```python
from build123d import *

# Parameters (mm, degrees)
F0_W     = 25
F0_H     = 16
F1_DEPTH = 4
F3_D     = 4.2
F3_DEPTH = 14.4
F3_TIP   = 1.2618073
F5_D     = 2.4
F5_DEPTH = 9.8
F5_TIP   = 0.7210327428


with BuildPart() as f1:
    # F0 (on Front) → F1 (new body, symmetric)
    with BuildSketch(Plane.XZ):
        Rectangle(F0_W, F0_H)
    extrude(amount=F1_DEPTH, both=True)

    # F3
    with Locations(Plane.XZ.offset(4)):
        with Locations((4.5, 2)):
            Hole(F3_D / 2, depth=F3_DEPTH)
            with Locations((0, 0, -(F3_DEPTH + F3_TIP / 2))):  # 118° drill point
                Cone(0, F3_D / 2, F3_TIP, mode=Mode.SUBTRACT)

    # F5
    with Locations(Plane.XY.offset(8)):
        with Locations((-0.5, 0), (-7.5, 0)):
            Hole(F5_D / 2, depth=F5_DEPTH)
            with Locations((0, 0, -(F5_DEPTH + F5_TIP / 2))):  # 118° drill point
                Cone(0, F5_D / 2, F5_TIP, mode=Mode.SUBTRACT)


solid = f1.part
```
Work out the finished part from the listing and answer in its coordinate system (mm). A direction names the side the tool comes from. Round coordinates to 2 decimals unless told otherwise and drop trailing zeros. Write each loop counter-clockwise with the first axis right and the second up, starting at its lowest first coordinate (ties: lowest second). Pieces come first, ordered by that corner, then holes. Notation, with made-up numbers: (0, -32.75) - (11, -32.75) arc R29 ccw to (11, -4.75) - close; hole circle Ø11 at (-27.75, 7). An arc over 180 degrees is marked (long way). Return JSON: item names as keys, results as strings. Group by question number.
Q1. The part is cut by section C-C on y = -2. Write down the section's boundary in (x, z), then the cut area to 3 significant figures.
Q2. The mould has two halves that part along X. Classify faces 3 (the flat face through (0, 4, 0)), 4 (the flat face through (12.5, 0, 0)), 5 (the cylindrical face through (4.96, 0.06, -0.05)), 6 (the conical face through (-0.665, -0.127, -2.396)): released by +X, released by -X, zero draft, split by the parting line, or undercut.
Q3. Find the intervals of material crossed by L1, parallel to X at y = 0, z = 1.25; L2, parallel to X at y = 0, z = 1.75; L3, parallel to Y at x = -7.5, z = 5, in increasing order.
Q4. The part is cut by section A-A on z = 2. Write down the section's boundary in (x, y).
Q5. For faces 1 (the flat face through (0, 2, 8)), 2 (the cylindrical face through (0.7, 0.05, 3.03)), determine the directions among +Z, -Z, +X, -X, +Y, -Y from which every point of the face is accessible in a straight line to the end or side of a thin tool.
Q6. The part is cut by section D-D on z = -0.75. Write down the section's boundary in (x, y), then the cut area to 3 significant figures.
Q7. Each of these flat-tipped pins is pushed along its axis until it touches: pin 1 Ø3.5 at (x, z) = (4.5, 2) entering from +Y; pin 2 Ø2 at (x, z) = (3, 2) entering from +Y. Where does it stop, or does it pass through?
Q8. The part is cut by section B-B on x = 4.5. Write down the section's boundary in (y, z), then the cut area to 3 significant figures.
Solved:
{
 "1": {"outline": "(-12.5, -8) - (12.5, -8) - (12.5, 8) - (-12.5, 8) - close; hole circle Ø4.2 at (4.5, 2)", "area": "386 mm²"},
 "2": {"face 3": "zero draft", "face 4": "released by +X", "face 5": "undercut", "face 6": "undercut"},
 "3": {"L1": "-12.5 to -8.7, -6.3 to -1.7, 0.7 to 2.54, 6.46 to 12.5", "L2": "-12.5 to -8.7, -6.3 to -1.7, 0.7 to 2.41, 6.59 to 12.5", "L3": "-4 to -1.2, 1.2 to 4"},
 "4": {"outline": "(-12.5, -4) - (2.4, -4) - (2.4, 4) - (-12.5, 4) - close; (6.6, -4) - (12.5, -4) - (12.5, 4) - (6.6, 4) - close; hole circle Ø2.4 at (-7.5, 0); hole circle Ø2.4 at (-0.5, 0)"},
 "5": {"face 1": "+Z, +X, -X, +Y, -Y", "face 2": "+Z"},
 "6": {"outline": "(-12.5, -4) - (12.5, -4) - (12.5, 4) - (-12.5, 4) - close; hole circle Ø2.4 at (-7.5, 0); hole circle Ø2.4 at (-0.5, 0)", "area": "191 mm²"},
 "7": {"pin 1": "through", "pin 2": "y = 4"},
 "8": {"outline": "(-4, -8) - (4, -8) - (4, -0.1) - (-4, -0.1) - close; (-4, 4.1) - (4, 4.1) - (4, 8) - (-4, 8) - close", "area": "94.4 mm²"}
}
